from build123d import *

# Parameters (mm, degrees)
SKETCH1_W           = 70
SKETCH1_H           = 110
SKETCH1_R           = 1.5
SKETCH1_R_2         = 2.4
BOSS_EXTRUDE1_DEPTH = 5
FILLET1_R           = 5


with BuildPart() as part:
    # Sketch1 → Boss-Extrude1 (new body)
    with BuildSketch(Plane.XY):
        Rectangle(SKETCH1_W, SKETCH1_H)
        with Locations((25, 42)):
            Circle(SKETCH1_R, mode=Mode.SUBTRACT)
        with Locations((25, -33)):
            Circle(SKETCH1_R, mode=Mode.SUBTRACT)
        with Locations((25, 32)):
            Circle(SKETCH1_R_2, mode=Mode.SUBTRACT)
        with Locations((25, -43)):
            Circle(SKETCH1_R_2, mode=Mode.SUBTRACT)
        with Locations((-22, 48)):
            Circle(SKETCH1_R, mode=Mode.SUBTRACT)
        with Locations((-22, -35)):
            Circle(SKETCH1_R, mode=Mode.SUBTRACT)
    extrude(amount=BOSS_EXTRUDE1_DEPTH)

    # Fillet1
    fillet1_edges = [part.edges().sort_by_distance(p)[0] for p in [
        (35, -55, 2.5),
        (-35, -55, 2.5),
        (-35, 55, 2.5),
        (35, 55, 2.5),
    ]]
    fillet(fillet1_edges, radius=FILLET1_R)


solid = part.part
Part model, mm, in its own coordinate system. Coordinates: 2 decimals unless noted, no trailing zeros. Loops run counter-clockwise (first coordinate to the right, second up) from the corner with the lowest first, then second, coordinate; pieces in that order, holes last. Notation, with made-up numbers: (39.25, -17.75) - (62.25, -17.75) arc R17 ccw to (62.25, 8.25) - close; hole circle Ø2 at (73.25, -31.5). An arc over 180 degrees is marked (long way). Write each question's results on one line, items separated by ' | '. Start each with the question number.
Q1. Two-plate mould, pull along X, no slides. Class faces 1 (the flat face through (-35, -1, 2)), 2 (the flat face through (0, 1, 5)), 3 (the cylindrical face through (26.11, -45.13, 2.46)): +X half, -X half, draft (parallel to the pull), parting line (faces both ways), or undercut.
Q2. Slice it at A-A on y = -43. Give the cut face in (x, z), and give its area (3 significant figures).
Q3. Slice it at B-B on x = -22. Give the cut face in (y, z), and give its area (3 significant figures).
Q4. Probe line 1 along Y through (x, z) = (-22, 1.8); line 2 along Y through (x, z) = (25, 1.8); line 3 along X through (y, z) = (50.5, 3.2). List the from-to ranges inside material, lowest first.
Q5. Slice it at C-C on y = 48. Give the cut face in (x, z).
Answer:
1) face 1: -X half | face 2: draft | face 3: undercut
2) outline: (-35, 0) - (22.6, 0) - (22.6, 5) - (-35, 5) - close; (27.4, 0) - (35, 0) - (35, 5) - (27.4, 5) - close | area: 326 mm2
3) outline: (-55, 0) - (-36.5, 0) - (-36.5, 5) - (-55, 5) - close; (-33.5, 0) - (46.5, 0) - (46.5, 5) - (-33.5, 5) - close; (49.5, 0) - (55, 0) - (55, 5) - (49.5, 5) - close | area: 520 mm2
4) line 1: y = -55 to -36.5, -33.5 to 46.5, 49.5 to 55 | line 2: y = -55 to -45.4, -40.6 to -34.5, -31.5 to 29.6, 34.4 to 40.5, 43.5 to 55 | line 3: x = -34.97 to 34.97
5) outline: (-35, 0) - (-23.5, 0) - (-23.5, 5) - (-35, 5) - close; (-20.5, 0) - (35, 0) - (35, 5) - (-20.5, 5) - close
